```python
from build123d import *

# Parameters (mm, degrees)
SKETCH1_R            = 2.265
BOSS_EXTRUDE1_DEPTH  = 3
SKETCH2_W            = 6.5
SKETCH2_H            = 20
CUT_EXTRUDE1_DEPTH   = 3
BOSS_EXTRUDE2_DEPTH  = 3
CUT_EXTRUDE2_DEPTH   = 3
SKETCH5_W            = 3
SKETCH5_H            = 26
BOSS_EXTRUDE6_DEPTH  = 3
FILLET1_R            = 1
SKETCH9_W            = 57
SKETCH9_H            = 3
CUT_EXTRUDE4_DEPTH   = 3
SKETCH11_W           = 21.1
SKETCH11_H           = 54
CUT_EXTRUDE6_DEPTH   = 3
SKETCH12_W           = 5.606838984
SKETCH12_H           = 3.16637745
CUT_EXTRUDE7_DEPTH   = 3
SKETCH14_W           = 13
SKETCH14_H           = 14
SKETCH14_W_2         = 11
SKETCH14_H_2         = 12
BOSS_EXTRUDE9_DEPTH  = 3
SKETCH15_W           = 1
SKETCH15_H           = 8.5
CUT_EXTRUDE8_DEPTH   = 3
SKETCH16_W           = 3.5
SKETCH16_H           = 8
BOSS_EXTRUDE10_DEPTH = 3
SKETCH17_W           = 1.5
SKETCH17_H           = 6
BOSS_EXTRUDE11_DEPTH = 3
CUT_EXTRUDE9_DEPTH   = 3
SKETCH19_W           = 2.1
SKETCH19_H           = 2
CUT_EXTRUDE10_DEPTH  = 3
BOSS_EXTRUDE16_DEPTH = 3
FILLET2_R            = 1
FILLET3_R            = 0.5
FILLET4_R            = 0.5
FILLET6_R            = 1
SKETCH21_W           = 8
SKETCH21_H           = 22
BOSS_EXTRUDE13_DEPTH = 3
SKETCH24_W           = 4
SKETCH24_H           = 6.433647318
CUT_EXTRUDE12_DEPTH  = 3
FILLET9_R            = 1
SKETCH25_W           = 4.5
SKETCH25_H           = 3.5
SKETCH25_W_2         = 4
SKETCH25_H_2         = 4
CUT_EXTRUDE14_DEPTH  = 3
SKETCH26_W           = 4
SKETCH26_H           = 2.433647318
BOSS_EXTRUDE15_DEPTH = 3
SKETCH27_W           = 3
SKETCH27_H           = 8.5
CUT_EXTRUDE15_DEPTH  = 3
SKETCH28_W           = 1.8
SKETCH28_H           = 4.5
CUT_EXTRUDE16_DEPTH  = 3
SKETCH29_W           = 1.997350186
SKETCH29_H           = 9.968253882
CUT_EXTRUDE17_DEPTH  = 3
SKETCH30_W           = 7.5
SKETCH30_H           = 1
CUT_EXTRUDE18_DEPTH  = 3
FILLET11_R           = 0.3
FILLET12_R           = 0.6
FILLET13_R           = 0.3


with BuildPart() as part:
    # Sketch1 → Boss-Extrude1 (new body)
    with BuildSketch(Plane(origin=(0, 0, 0), x_dir=(1, 0, 0), z_dir=(0, 1, 0))):
        with BuildLine():
            Line((0, -4.265), (0, -58.735))
            ThreePointArc((0, -58.735), (-3.015810422, -66.015810422), (4.265, -63))
            Line((4.265, -63), (87.735, -63))
            ThreePointArc((87.735, -63), (95.015810422, -66.015810422), (92, -58.735))
            Line((92, -58.735), (92, -4.265))
            ThreePointArc((92, -4.265), (95.015810422, 3.015810422), (87.735, 0))
            Line((87.735, 0), (4.265, 0))
            ThreePointArc((4.265, 0), (-3.015810422, 3.015810422), (0, -4.265))
        make_face()
        with Locations(Location((0, 0, 0), (0, 0, 270))):
            Circle(SKETCH1_R, mode=Mode.SUBTRACT)
        with Locations(Location((92, 0, 0), (0, 0, 270))):
            Circle(SKETCH1_R, mode=Mode.SUBTRACT)
        with Locations(Location((92, -63, 0), (0, 0, 270))):
            Circle(SKETCH1_R, mode=Mode.SUBTRACT)
        with Locations(Location((0, -63, 0), (0, 0, 270))):
            Circle(SKETCH1_R, mode=Mode.SUBTRACT)
    extrude(amount=BOSS_EXTRUDE1_DEPTH)

    # Sketch2 → Cut-Extrude1 (cut)
    with BuildSketch(Plane(origin=(0, 3, 0), x_dir=(1, 0, 0), z_dir=(0, 1, 0))):
        with Locations((3.25, -31.5)):
            Rectangle(SKETCH2_W, SKETCH2_H)
    extrude(amount=-CUT_EXTRUDE1_DEPTH, mode=Mode.SUBTRACT)

    # Sketch3 → Boss-Extrude2 (add)
    with BuildSketch(Plane(origin=(0, 3, 0), x_dir=(1, 0, 0), z_dir=(0, 1, 0))):
        with BuildLine():
            Line((-2.7, -15.5), (0, -14.9))
            Line((0, -14.9), (0, -21.5))
            Line((0, -21.5), (-2.5, -21.5))
            ThreePointArc((-2.5, -21.5), (-2.853553391, -21.353553391), (-3, -21))
            Line((-3, -21), (-3, -15.8))
            ThreePointArc((-3, -15.8), (-2.912132034, -15.587867966), (-2.7, -15.5))
        make_face()
        with BuildLine():
            Line((-3, -42), (-3, -47.2))
            ThreePointArc((-3, -47.2), (-2.912132034, -47.412132034), (-2.7, -47.5))
            Line((-2.7, -47.5), (0, -48.1))
            Line((0, -48.1), (0, -41.5))
            Line((0, -41.5), (-2.5, -41.5))
            ThreePointArc((-2.5, -41.5), (-2.853553391, -41.646446609), (-3, -42))
        make_face()
    extrude(amount=-BOSS_EXTRUDE2_DEPTH)

    # Sketch6 → Cut-Extrude2 (cut)
    with BuildSketch(Plane(origin=(0, 3, 0), x_dir=(1, 0, 0), z_dir=(0, 1, 0))):
        with BuildLine():
            Line((5, -3), (65.9, -3))
            ThreePointArc((65.9, -3), (68.021320344, -3.878679656), (68.9, -6))
            Line((68.9, -6), (68.9, -57))
            ThreePointArc((68.9, -57), (68.021320344, -59.121320344), (65.9, -60))
            Line((65.9, -60), (5, -60))
            ThreePointArc((5, -60), (2.878679656, -59.121320344), (2, -57))
            Line((2, -57), (2, -6))
            ThreePointArc((2, -6), (2.878679656, -3.878679656), (5, -3))
        make_face()
    extrude(amount=-CUT_EXTRUDE2_DEPTH, mode=Mode.SUBTRACT)

    # Sketch5 → Boss-Extrude6 (add)
    with BuildSketch(Plane(origin=(0, 3, 0), x_dir=(1, 0, 0), z_dir=(0, 1, 0))):
        with Locations((1.5, -32.5825)):
            Rectangle(SKETCH5_W, SKETCH5_H)
    extrude(amount=-BOSS_EXTRUDE6_DEPTH)

    # Fillet1
    fillet1_edges = [part.edges().sort_by_distance(p)[0] for p in [
        (3, 1.5, 45.5825),
        (3, 1.5, 19.5825),
    ]]
    fillet(fillet1_edges, radius=FILLET1_R - 0.0001)  # a hair under: the kernel refuses the full size

    # Sketch9 → Cut-Extrude4 (cut)
    with BuildSketch(Plane(origin=(0, 3, 0), x_dir=(1, 0, 0), z_dir=(0, 1, 0))):
        with Locations((36.5, -61.5)):
            Rectangle(SKETCH9_W, SKETCH9_H)
    extrude(amount=-CUT_EXTRUDE4_DEPTH, mode=Mode.SUBTRACT)

    # Sketch11 → Cut-Extrude6 (cut)
    with BuildSketch(Plane(origin=(0, 3, 0), x_dir=(1, 0, 0), z_dir=(0, 1, 0))):
        with Locations((81.45, -32.5)):
            Rectangle(SKETCH11_W, SKETCH11_H)
    extrude(amount=-CUT_EXTRUDE6_DEPTH, mode=Mode.SUBTRACT)

    # Sketch12 → Cut-Extrude7 (cut)
    with BuildSketch(Plane(origin=(0, 3, 0), x_dir=(1, 0, 0), z_dir=(0, 1, 0))):
        with Locations((94.803419492, -57.916811275)):
            Rectangle(SKETCH12_W, SKETCH12_H)
    extrude(amount=-CUT_EXTRUDE7_DEPTH, mode=Mode.SUBTRACT)

    # Sketch14 → Boss-Extrude9 (add)
    with BuildSketch(Plane(origin=(0, 3, 0), x_dir=(1, 0, 0), z_dir=(0, 1, 0))):
        with Locations((62.4, -24)):
            Rectangle(SKETCH14_W, SKETCH14_H)
        with Locations((62.4, -24)):
            Rectangle(SKETCH14_W_2, SKETCH14_H_2, mode=Mode.SUBTRACT)
    extrude(amount=-BOSS_EXTRUDE9_DEPTH)

    # Sketch15 → Cut-Extrude8 (cut)
    with BuildSketch(Plane(origin=(0, 3, 0), x_dir=(1, 0, 0), z_dir=(0, 1, 0))):
        with Locations((70.4, -27.25)):
            Rectangle(SKETCH15_W, SKETCH15_H)
    extrude(amount=-CUT_EXTRUDE8_DEPTH, mode=Mode.SUBTRACT)

    # Sketch16 → Boss-Extrude10 (add)
    with BuildSketch(Plane(origin=(0, 3, 0), x_dir=(1, 0, 0), z_dir=(0, 1, 0))):
        with Locations((72.65, -35.5)):
            Rectangle(SKETCH16_W, SKETCH16_H)
    extrude(amount=-BOSS_EXTRUDE10_DEPTH)

    # Sketch17 → Boss-Extrude11 (add)
    with BuildSketch(Plane(origin=(0, 3, 0), x_dir=(1, 0, 0), z_dir=(0, 1, 0))):
        with Locations((67.15, -21)):
            Rectangle(SKETCH17_W, SKETCH17_H)
    extrude(amount=-BOSS_EXTRUDE11_DEPTH)

    # Sketch18 → Cut-Extrude9 (cut)
    with BuildSketch(Plane(origin=(0, 3, 0), x_dir=(1, 0, 0), z_dir=(0, 1, 0))):
        with BuildLine():
            Line((66.716936581, -18.590391311), (67.692016523, -17.197832836))
            ThreePointArc((67.692016523, -17.197832836), (67.75656691, -17.156709704), (67.831289371, -17.173275275))
            Line((67.831289371, -17.173275275), (70.534491117, -19.066077515))
            ThreePointArc((70.534491117, -19.066077515), (70.575614249, -19.130627902), (70.559048678, -19.205350363))
            Line((70.559048678, -19.205350363), (69.583968736, -20.597908838))
            ThreePointArc((69.583968736, -20.597908838), (69.51941835, -20.63903197), (69.444695888, -20.622466399))
            Line((69.444695888, -20.622466399), (66.741494142, -18.729664159))
            ThreePointArc((66.741494142, -18.729664159), (66.70037101, -18.665113772), (66.716936581, -18.590391311))
        make_face()
        with BuildLine():
            Line((66.501627394, -21.606320712), (67.591422623, -20.049931828))
            ThreePointArc((67.591422623, -20.049931828), (67.65597301, -20.008808696), (67.730695471, -20.025374267))
            Line((67.730695471, -20.025374267), (70.433897217, -21.918176507))
            ThreePointArc((70.433897217, -21.918176507), (70.475020349, -21.982726894), (70.458454778, -22.057449355))
            Line((70.458454778, -22.057449355), (69.368659549, -23.613838239))
            ThreePointArc((69.368659549, -23.613838239), (69.304109162, -23.654961371), (69.229386701, -23.6383958))
            Line((69.229386701, -23.6383958), (66.526184955, -21.74559356))
            ThreePointArc((66.526184955, -21.74559356), (66.485061823, -21.681043173), (66.501627394, -21.606320712))
        make_face()
    extrude(amount=-CUT_EXTRUDE9_DEPTH, mode=Mode.SUBTRACT)

    # Sketch19 → Cut-Extrude10 (cut)
    with BuildSketch(Plane(origin=(0, 3, 0), x_dir=(1, 0, 0), z_dir=(0, 1, 0))):
        with Locations((56.95, -30)):
            Rectangle(SKETCH19_W, SKETCH19_H)
    extrude(amount=-CUT_EXTRUDE10_DEPTH, mode=Mode.SUBTRACT)

    # Sketch31 → Boss-Extrude16 (add)
    with BuildSketch(Plane(origin=(0, 3, 0), x_dir=(1, 0, 0), z_dir=(0, 1, 0))):
        Polygon((58, -30), (59.5, -30), (59.5, -28.5), (58, -28.5), (56.9, -28.5), (56.9, -29), (58, -29), align=None)
    extrude(amount=-BOSS_EXTRUDE16_DEPTH)

    # Fillet2
    fillet2_edges = [part.edges().sort_by_distance(p)[0] for p in [
        (68.9, 1.5, 31),
        (55.9, 1.5, 17),
        (55.9, 1.5, 29),
        (58, 1.5, 31),
    ]]
    fillet(fillet2_edges, radius=FILLET2_R)

    # Fillet3
    fillet3_edges = [part.edges().sort_by_distance(p)[0] for p in [
        (68.9, 1.5, 17),
    ]]
    fillet(fillet3_edges, radius=FILLET3_R)

    # Fillet4
    fillet4_edges = [part.edges().sort_by_distance(p)[0] for p in [
        (58, 1.5, 29),
    ]]
    fillet(fillet4_edges, radius=FILLET4_R)

    # Fillet6
    fillet6_edges = [part.edges().sort_by_distance(p)[0] for p in [
        (74.4, 1.5, 31.5),
        (74.4, 1.5, 39.5),
    ]]
    fillet(fillet6_edges, radius=FILLET6_R)

    # Sketch21 → Boss-Extrude13 (add)
    with BuildSketch(Plane(origin=(0, 3, 0), x_dir=(1, 0, 0), z_dir=(0, 1, 0))):
        with Locations((66.4, -52)):
            Rectangle(SKETCH21_W, SKETCH21_H)
    extrude(amount=-BOSS_EXTRUDE13_DEPTH)

    # Sketch24 → Cut-Extrude12 (cut)
    with BuildSketch(Plane(origin=(0, 3, 0), x_dir=(1, 0, 0), z_dir=(0, 1, 0))):
        with Locations((70.14, -48.716823659)):
            Rectangle(SKETCH24_W, SKETCH24_H)
    extrude(amount=-CUT_EXTRUDE12_DEPTH, mode=Mode.SUBTRACT)

    # Fillet9
    fillet9_edges = [part.edges().sort_by_distance(p)[0] for p in [
        (70.9, 1.5, 45.5),
    ]]
    fillet(fillet9_edges, radius=FILLET9_R)

    # Sketch25 → Cut-Extrude14 (cut)
    with BuildSketch(Plane(origin=(0, 3, 0), x_dir=(1, 0, 0), z_dir=(0, 1, 0))):
        with Locations((66.15, -43.25)):
            Rectangle(SKETCH25_W, SKETCH25_H)
        with Locations((68.9, -47.5)):
            Rectangle(SKETCH25_W_2, SKETCH25_H_2)
    extrude(amount=-CUT_EXTRUDE14_DEPTH, mode=Mode.SUBTRACT)

    # Sketch26 → Boss-Extrude15 (add)
    with BuildSketch(Plane(origin=(0, 3, 0), x_dir=(1, 0, 0), z_dir=(0, 1, 0))):
        with Locations((68.9, -50.716823659)):
            Rectangle(SKETCH26_W, SKETCH26_H)
    extrude(amount=-BOSS_EXTRUDE15_DEPTH)

    # Sketch27 → Cut-Extrude15 (cut)
    with BuildSketch(Plane(origin=(0, 3, 0), x_dir=(1, 0, 0), z_dir=(0, 1, 0))):
        with Locations((64.8, -49.75)):
            Rectangle(SKETCH27_W, SKETCH27_H)
    extrude(amount=-CUT_EXTRUDE15_DEPTH, mode=Mode.SUBTRACT)

    # Sketch28 → Cut-Extrude16 (cut)
    with BuildSketch(Plane(origin=(0, 3, 0), x_dir=(1, 0, 0), z_dir=(0, 1, 0))):
        with Locations((67.5, -52.05)):
            Rectangle(SKETCH28_W, SKETCH28_H)
    extrude(amount=-CUT_EXTRUDE16_DEPTH, mode=Mode.SUBTRACT)

    # Sketch29 → Cut-Extrude17 (cut)
    with BuildSketch(Plane(origin=(0, 3, 0), x_dir=(1, 0, 0), z_dir=(0, 1, 0))):
        with Locations((69.901324907, -54.484126941)):
            Rectangle(SKETCH29_W, SKETCH29_H)
    extrude(amount=-CUT_EXTRUDE17_DEPTH, mode=Mode.SUBTRACT)

    # Sketch30 → Cut-Extrude18 (cut)
    with BuildSketch(Plane(origin=(0, 3, 0), x_dir=(1, 0, 0), z_dir=(0, 1, 0))):
        with Locations((66.15, -62.5)):
            Rectangle(SKETCH30_W, SKETCH30_H)
    extrude(amount=-CUT_EXTRUDE18_DEPTH, mode=Mode.SUBTRACT)

    # Fillet11
    fillet11_edges = [part.edges().sort_by_distance(p)[0] for p in [
        (69.9, 1.5, 62),
    ]]
    fillet(fillet11_edges, radius=FILLET11_R)

    # Fillet12
    fillet12_edges = [part.edges().sort_by_distance(p)[0] for p in [
        (92, 1.5, 4.265),
    ]]
    fillet(fillet12_edges, radius=FILLET12_R)

    # Fillet13
    fillet13_edges = [part.edges().sort_by_distance(p)[0] for p in [
        (92, 1.5, 5.5),
    ]]
    fillet(fillet13_edges, radius=FILLET13_R)


solid = part.part
```
CAD build for the part. Positions are in the model's coordinates, mm. A direction names the side the tool comes from. Give positions to 0.01 mm unless a question says otherwise; leave off trailing zeros. Loops run counter-clockwise (first coordinate to the right, second up) from the corner with the lowest first, then second, coordinate; pieces in that order, holes last. Notation, with made-up numbers: M -39,38 L -19,38 A19 cw -19,63 Z; hole C -27,-39.75 d2. An arc over 180 degrees is marked long. Use one line per item in the form item = value.
Item 1: Slice it at C-C (y = 2.45). Count the separate pieces of the cut face and the enclosed holes in it, plus the area to 3 significant figures.
Determined:
separate_pieces = 1
enclosed_holes = 10
area = 949 mm2
Item 2: Drill centre lines: probe 1 along Z at (x, y) = (63, 1.4); probe 2 along X at (y, z) = (2, 50.5); probe 3 along X at (y, z) = (2.8, 10.5). Where is each one in solid material? Low to high. Write a range as from..to.
Determined:
probe_1 = 0..3, 17..18, 30..31, 41..62
probe_2 = 0..2, 62.4..63.3, 66.3..66.6, 68.4..68.9
probe_3 = 0..2, 68.9..70.9
Item 3: Two-plate mould, pull along X, no slides. Class faces 1 (the face through (56.9, 3, 28.7)), 2 (the face through (0, 2, 32)), 3 (the face through (63.3, 2, 50)): pulls with the +X half, pulls with the -X half, needs draft (parallel to the pull), parting line crosses it, or undercut.
Determined:
face_1 = needs draft
face_2 = pulls with the -X half
face_3 = undercut
Item 4: Which spindle directions (+Z, -Z, +X, -X, +Y, -Y) get a long thin tool onto all of the face, cutting with end or side? Do faces 4 (the face through (-1, 2, 41.5)), 5 (the face through (68.11, 1.52, 19.69)), 6 (the face through (68, 2, 45.5)). Say none if no direction does.
Determined:
face_4 = -X, +Y, -Y
face_5 = +Y, -Y
face_6 = +X, +Y, -Y
Item 5: Flat gauge pins, fed straight in: pin 1 (1.5 mm diameter, centred on y = 1.5, z = 35, fed in from +X); pin 2 (0.9 mm diameter, centred on x = 76.5, y = 1.5, fed in from +Z); pin 3 (0.9 mm diameter, centred on x = 67, y = 1, fed in from +Z); pin 4 (2.5 mm diameter, centred on x = 92, z = 63, fed in from -Y) (3 decimals). Where does each tip first touch, or does it go through?
Determined:
pin_1 = 74.4
pin_2 = 63
pin_3 = 62
pin_4 = through
Item 6: Slice it at B-B (x = 15). List the corners of the cut face in (y, z), plus the area to 3 significant figures.
Determined:
outline = M 0,0 L 3,0 L 3,3 L 0,3 Z
area = 9.00 mm2
Item 7: Slice it at A-A (z = 26.5). List the corners of the cut face in (x, y).
Determined:
outline = M 0,0 L 3,0 L 3,3 L 0,3 Z; M 55.9,0 L 56.9,0 L 56.9,3 L 55.9,3 Z; M 67.9,0 L 69.9,0 L 69.9,3 L 67.9,3 Z
